```python
from build123d import *

# Parameters (mm, degrees)
PAD007_DEPTH    = 50
SKETCH009_R     = 10
POCKET001_DEPTH = 22.251
SKETCH010_R     = 11.25
POCKET002_DEPTH = 19.251
CHAMFER001_SIZE = 4


with BuildPart() as part:
    # Sketch008 (on Face1 of Binder002) → Pad007 (new body)
    with BuildSketch(Plane.XZ.offset(-29)):
        Polygon((37, 0), (37, 10), (-27.5, 10), (-27.5, 22.25), (-36, 22.25), (-36, 0), align=None)
    extrude(amount=PAD007_DEPTH)

    # Sketch009 → Pocket001 (cut, through all)
    with BuildSketch(Plane.XY):
        Circle(SKETCH009_R)
    extrude(amount=POCKET001_DEPTH, mode=Mode.SUBTRACT)

    # Sketch010 → Pocket002 (cut, through all)
    with BuildSketch(Plane.XY.offset(3)):
        Circle(SKETCH010_R)
    extrude(amount=POCKET002_DEPTH, mode=Mode.SUBTRACT)

    # Chamfer001
    chamfer001_edges = [part.edges().sort_by_distance(p)[0] for p in [
        (-31.75, -21, 22.25),
        (37, -21, 5),
        (-36, 4, 0),
        (0.5, -21, 0),
        (37, 4, 0),
    ]]
    chamfer(chamfer001_edges, length=CHAMFER001_SIZE)


solid = part.part
```
Part model, mm, in its own coordinate system. A direction names the side the tool comes from. Round coordinates to 2 decimals unless told otherwise and drop trailing zeros. Loops run counter-clockwise (first coordinate to the right, second up) from the corner with the lowest first, then second, coordinate; pieces in that order, holes last. Notation, with made-up numbers: (34, -20.5) -> (60, -20.5) arc R32 ccw to (60, 6.5) -> close; hole circle Ø1 at (84, -27). An arc over 180 degrees is marked (long way). Use CSV: the item, a comma, the result in double quotes. Start each with the question number.
1) Pull direction X, two halves, no side cores. Call faces 1 (the flat face through (-36, 4, 13)), 2 (the cylindrical face through (-2.17, -9.76, 1.48)), 3 (the flat face through (37, 6, 7)): +X half, -X half, draft (parallel to the pull), parting line (faces both ways), or undercut.
2) Drop flat-ended pins along their axis: P1, Ø13.5, axis at x = 0, y = 0, coming from the +Z side; P2, Ø3, axis at x = -4.5, y = 14.5, coming from the +Z side; P3, Ø11, axis at x = -2.5, y = 4, coming from the +Z side; P4, Ø10, axis at y = 4, z = 19, coming from the +X side. Give the stop position or say it passes through.
3) Cut at A-A, the plane y = 0. Write the cut outline in (x, z).
4) Cut at B-B, the plane x = 0. Write the cut outline in (y, z).
5) Wall check: L1, parallel to X at y = 0, z = 7.25; L2, parallel to Y at x = 0, z = 5; L3, parallel to Z at x = -1.5, y = 18. Give the ranges that are in metal, low to high. Write a range as [from, to].
6) Cut at C-C, the plane y = 15. Write the cut outline in (x, z), plus the area to 3 significant figures.
7) Cut at D-D, the plane z = 20.5. Write the cut outline in (x, y), plus the area to 3 significant figures.
8) Which spindle directions (+Z, -Z, +X, -X, +Y, -Y) get a long thin tool onto all of the face, cutting with end or side? Do faces 4 (the flat face through (-8, -7, 3)), 5 (the flat face through (0, 11, 0)), 6 (the flat face through (12, 4, 10)). Say none if no direction does.
Determined:
1,face 1,"-X half"
1,face 2,"undercut"
1,face 3,"+X half"
2,P1,"passes through"
2,P2,"stops at z = 10"
2,P3,"stops at z = 3"
2,P4,"stops at x = -27.5"
3,outline,"(-36, 4) -> (-32, 0) -> (-10, 0) -> (-10, 3) -> (-11.25, 3) -> (-11.25, 10) -> (-27.5, 10) -> (-27.5, 22.25) -> (-36, 22.25) -> close; (10, 0) -> (33, 0) -> (37, 4) -> (37, 10) -> (11.25, 10) -> (11.25, 3) -> (10, 3) -> close"
4,outline,"(-21, 4) -> (-17, 0) -> (-10, 0) -> (-10, 3) -> (-11.25, 3) -> (-11.25, 10) -> (-21, 10) -> close; (10, 0) -> (29, 0) -> (29, 10) -> (11.25, 10) -> (11.25, 3) -> (10, 3) -> close"
5,L1,"x = [-36, -11.25], [11.25, 37]"
5,L2,"y = [-21, -11.25], [11.25, 29]"
5,L3,"z = [0, 10]"
6,outline,"(-36, 4) -> (-32, 0) -> (33, 0) -> (37, 4) -> (37, 10) -> (-27.5, 10) -> (-27.5, 22.25) -> (-36, 22.25) -> close"
6,area,"818 mm2"
7,outline,"(-36, -18.75) -> (-27.5, -18.75) -> (-27.5, 29) -> (-36, 29) -> close"
7,area,"406 mm2"
8,face 4,"+Z"
8,face 5,"-Z, +X, -X, +Y, -Y"
8,face 6,"+Z, +X, +Y, -Y"
